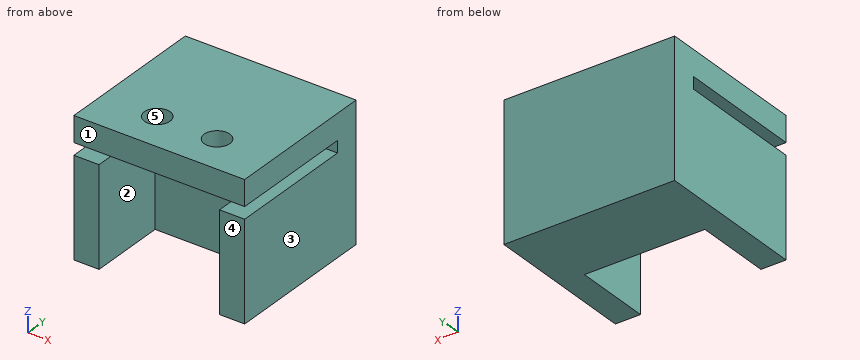
from build123d import *

# Parameters (mm, degrees)
CROQUIS1_W              = 20
CROQUIS1_H              = 18
SALIENTE_EXTRUIR1_DEPTH = 16
CROQUIS2_W              = 14.1
CROQUIS2_H              = 11.6
CORTAR_EXTRUIR1_DEPTH   = 9.05
CROQUIS4_W              = 20
CROQUIS4_H              = 1.4
CORTAR_EXTRUIR2_DEPTH   = 15
CROQUIS5_R              = 1.5
CORTAR_EXTRUIR3_DEPTH   = 17


with BuildPart() as part:
    # Croquis1 → Saliente-Extruir1 (new body)
    with BuildSketch(Plane.XY):
        Rectangle(CROQUIS1_W, CROQUIS1_H)
    extrude(amount=-SALIENTE_EXTRUIR1_DEPTH)

    # Croquis2 → Cortar-Extruir1 (cut)
    with BuildSketch(Plane.XZ.offset(9)):
        with Locations((0, -10.2)):
            Rectangle(CROQUIS2_W, CROQUIS2_H)
    extrude(amount=-CORTAR_EXTRUIR1_DEPTH, mode=Mode.SUBTRACT)

    # Croquis4 → Cortar-Extruir2 (cut)
    with BuildSketch(Plane.XZ.offset(9)):
        with Locations((0, -3.7)):
            Rectangle(CROQUIS4_W, CROQUIS4_H)
    extrude(amount=-CORTAR_EXTRUIR2_DEPTH, mode=Mode.SUBTRACT)

    # Croquis5 → Cortar-Extruir3 (cut, through all)
    with BuildSketch(Plane.XY):
        with Locations((-3.5, -4.5)):
            Circle(CROQUIS5_R)
        with Locations((3.5, -4.5)):
            Circle(CROQUIS5_R)
    extrude(amount=-CORTAR_EXTRUIR3_DEPTH, mode=Mode.SUBTRACT)


solid = part.part
Part model, mm, in its own coordinate system. Face numbers are marked on the shaded views. A direction names the side the tool comes from. Round coordinates to 2 decimals unless told otherwise and drop trailing zeros. Write each loop counter-clockwise with the first axis right and the second up, starting at its lowest first coordinate (ties: lowest second). Pieces come first, ordered by that corner, then holes. Notation, with made-up numbers: (22, 64) - (38, 64) arc R10 cw to (38, 80) - close; hole circle Ø11 at (13, 76.5). An arc over 180 degrees is marked (long way). Use CSV: the item, a comma, the result in double quotes.
Item 1: Pull direction X, two halves, no side cores. Call the marked faces 3, 4 and 5: pulls with the +X half, pulls with the -X half, needs draft (parallel to the pull), parting line crosses it, or undercut.
Results list:
face 3,"pulls with the +X half"
face 4,"needs draft"
face 5,"undercut"
Item 2: Slice it at C-C, the plane y = -4.5. Write the cut outline in (x, z), then the cut area to 3 significant figures.
Results list:
outline,"(-10, -16) - (-7.05, -16) - (-7.05, -4.4) - (-10, -4.4) - close; (-10, -3) - (-5, -3) - (-5, 0) - (-10, 0) - close; (-2, -3) - (2, -3) - (2, 0) - (-2, 0) - close; (5, -3) - (10, -3) - (10, 0) - (5, 0) - close; (7.05, -16) - (10, -16) - (10, -4.4) - (7.05, -4.4) - close"
area,"110 mm²"
Item 3: Tool access for the marked faces 1 and 2: list every direction of +Z, -Z, +X, -X, +Y, -Y with a clear straight run to the whole face (end or side of a thin tool).
Results list:
face 1,"+Z, -Z, +X, -X, -Y"
face 2,"-Z, -Y"
Item 4: Slice it at A-A, the plane y = -2. Write the cut outline in (x, z), then the cut area to 3 significant figures.
Results list:
outline,"(-10, -16) - (-7.05, -16) - (-7.05, -4.4) - (-10, -4.4) - close; (-10, -3) - (10, -3) - (10, 0) - (-10, 0) - close; (7.05, -16) - (10, -16) - (10, -4.4) - (7.05, -4.4) - close"
area,"128 mm²"
Item 5: Flat gauge pins, fed straight in: P1, Ø7.5, axis at x = 2, y = -4, coming from the +Z side; P2, Ø8, axis at x = -2, z = -8.5, coming from the -Y side; P3, Ø2.5, axis at x = -3.5, y = -4.5, coming from the -Z side. Where does each tip first touch, or does it go through?
Results list:
P1,"stops at z = 0"
P2,"stops at y = 0.05"
P3,"passes through"
Item 6: Wall check: L1, parallel to Z at x = 3.25, y = 2.5; L2, parallel to X at y = -7.25, z = -13.75; L3, parallel to Y at x = -3.5, z = -1.9. Give the ranges that are in metal, low to high.
Results list:
L1,"z = -16 to -4.4, -3 to 0"
L2,"x = -10 to -7.05, 7.05 to 10"
L3,"y = -9 to -6, -3 to 9"
Item 7: Slice it at B-B, the plane x = -3.5. Write the cut outline in (y, z), then the cut area to 3 significant figures.
Results list:
outline,"(-9, -3) - (-6, -3) - (-6, 0) - (-9, 0) - close; (-3, -3) - (6, -3) - (6, -4.4) - (0.05, -4.4) - (0.05, -16) - (9, -16) - (9, 0) - (-3, 0) - close"
area,"153 mm²"
Item 8: Slice it at D-D, the plane y = 4. Write the cut outline in (x, z), then the cut area to 3 significant figures.
Results list:
outline,"(-10, -16) - (10, -16) - (10, -4.4) - (-10, -4.4) - close; (-10, -3) - (10, -3) - (10, 0) - (-10, 0) - close"
area,"292 mm²"
